Here's how the part is built. I have some questions about the finished solid (model axes, mm). Face numbers are marked on the shaded views. A direction names the side the tool comes from. Give positions to 0.01 mm unless a question says otherwise; leave off trailing zeros. Loops run counter-clockwise (first coordinate to the right, second up) from the corner with the lowest first, then second, coordinate; pieces in that order, holes last.
Q1. Suppose I cut it at B-B (y = 0). List the corners of the cut face in (x, z) for me.
Q2. For the marked faces 1 and 2, which set-ups out of +Z, -Z, +X, -X, +Y, -Y let a thin tool reach every point of the face, with its end or its side?
Q3. Suppose I cut it at A-A (x = 0). List the corners of the cut face in (y, z) for me.
Q4. Suppose I cut it at D-D (z = -20). List the corners of the cut face in (x, y) for me.
Q5. I need wall thicknesses on probe 1 along Z at (x, y) = (2, -3.75); probe 2 along Z at (x, y) = (-3, -1.75); probe 3 along X at (y, z) = (0.75, -13.5). Which ranges of each line are inside material? Lowest first, please.
Q6. I'm going to push flat-ended pins straight in: P1, Ø2, axis at y = -1.5, z = -14.5, coming from the +X side; P2, Ø6, axis at y = 4.5, z = -11.5, coming from the +X side; P3, Ø3, axis at x = -2.5, z = -7, coming from the +Y side. Where does each tip first touch, or does it pass through?
Q7. Suppose I cut it at C-C (z = -4.5). List the corners of the cut face in (x, y) for me, and give its area (3 significant figures).
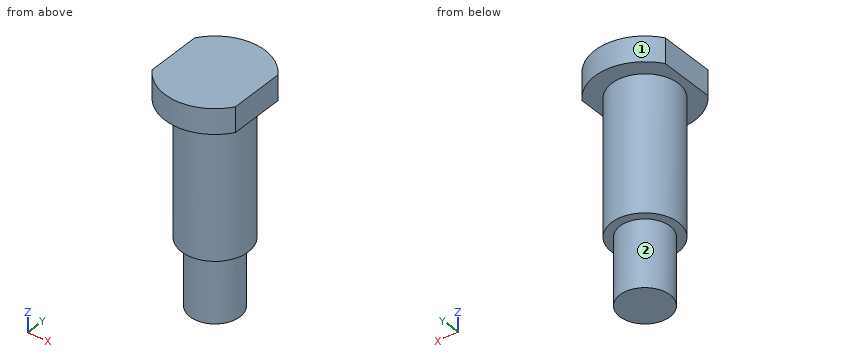
```python
from build123d import *

# Parameters (mm, degrees)
SKETCH_3_OUTSIDE_W   = 20.412
SKETCH_3_OUTSIDE_H   = 20.412
SKETCH_3_OUTSIDE_W_2 = 10
SKETCH_3_OUTSIDE_H_2 = 13.079471602
CUT_EXTRUDE_1_DEPTH  = 10


with BuildPart() as part:
    # 草图2 → 旋转1 (revolve)
    with BuildSketch(Plane(origin=(0, 0, 0), x_dir=(0, 0, -1), z_dir=(1, 0, 0))):
        Polygon((0, 0), (0, 6), (3, 6), (3, 4), (19.2, 4), (19.2, 3), (27.2, 3), (27.2, 0), align=None)
    revolve(axis=Axis((0, 0, 0), (0, 0, -1)))

    # 草图3 outside → 切除-拉伸1 (cut)
    with BuildSketch(Plane.XY):
        Rectangle(SKETCH_3_OUTSIDE_W, SKETCH_3_OUTSIDE_H)
        Rectangle(SKETCH_3_OUTSIDE_W_2, SKETCH_3_OUTSIDE_H_2, mode=Mode.SUBTRACT)
    extrude(amount=-CUT_EXTRUDE_1_DEPTH, mode=Mode.SUBTRACT)


solid = part.part
```
Solutions:
1. outline: (-5, -3) - (-4, -3) - (-4, -19.2) - (-3, -19.2) - (-3, -27.2) - (3, -27.2) - (3, -19.2) - (4, -19.2) - (4, -3) - (5, -3) - (5, 0) - (-5, 0) - close
2. face 1: +Z, -Z, +Y
2. face 2: -Z
3. outline: (-6, -3) - (-4, -3) - (-4, -19.2) - (-3, -19.2) - (-3, -27.2) - (3, -27.2) - (3, -19.2) - (4, -19.2) - (4, -3) - (6, -3) - (6, 0) - (-6, 0) - close
4. outline: circle Ø6 at (0, 0)
5. probe 1: z = -3 to 0
5. probe 2: z = -19.2 to 0
5. probe 3: x = -3.93 to 3.93
6. P1: stops at x = 3.97
6. P2: stops at x = 3.71
6. P3: stops at y = 3.87
7. outline: circle Ø8 at (0, 0)
7. area: 50.3 mm2
